Verification items for this drawing (mm, ordinates from the low corner). Round coordinates to 2 decimals unless told otherwise and drop trailing zeros. Order: outer loops, then holes, each group sorted by start corner. A loop starts at its lowest first (then second) coordinate and runs counter-clockwise, first axis right, second up. Notation, with made-up numbers: (49.25, 69) -> (87.25, 69) arc R18 ccw to (87.25, 87) -> close; hole circle Ø3 at (27, -13). An arc over 180 degrees is marked (long way). Answer in a Markdown table with one row per item. Add a question column.
1. Material ranges on L1, parallel to X at y = 48.5, z = 12; L2, parallel to Z at x = 12.25, y = 77.5; L3, parallel to X at y = 8, z = 9.5, recorded low to high. Write a range as from..to.
2. Sectioned sample at A-A, the plane x = 12.7. Record the boundary of the cut face in (y, z) (1 decimal).
3. Depth check by flat-ended pin: P1, Ø5, axis at x = 22, y = 36.5, coming from the -Z side; P2, Ø3, axis at x = 11, y = 64, coming from the +Z side; P3, Ø1, axis at y = 59.5, z = 14, coming from the +X side. Enter the tip coordinate at first touch or a pass-through.
4. Sectioned sample at D-D, the plane z = 20.75. Record the boundary of the cut face in (x, y).
5. Sectioned sample at B-B, the plane z = 12.7. Record the boundary of the cut face in (x, y) (1 decimal).
6. Sectioned sample at C-C, the plane x = 19.75. Record the boundary of the cut face in (y, z) (1 decimal), then the cut area to 3 significant figures.
7. Draft check along Z on the marked faces 1 and 2. Enter one of: +Z half, -Z half, draft (parallel to the pull), parting line (faces both ways), or undercut.
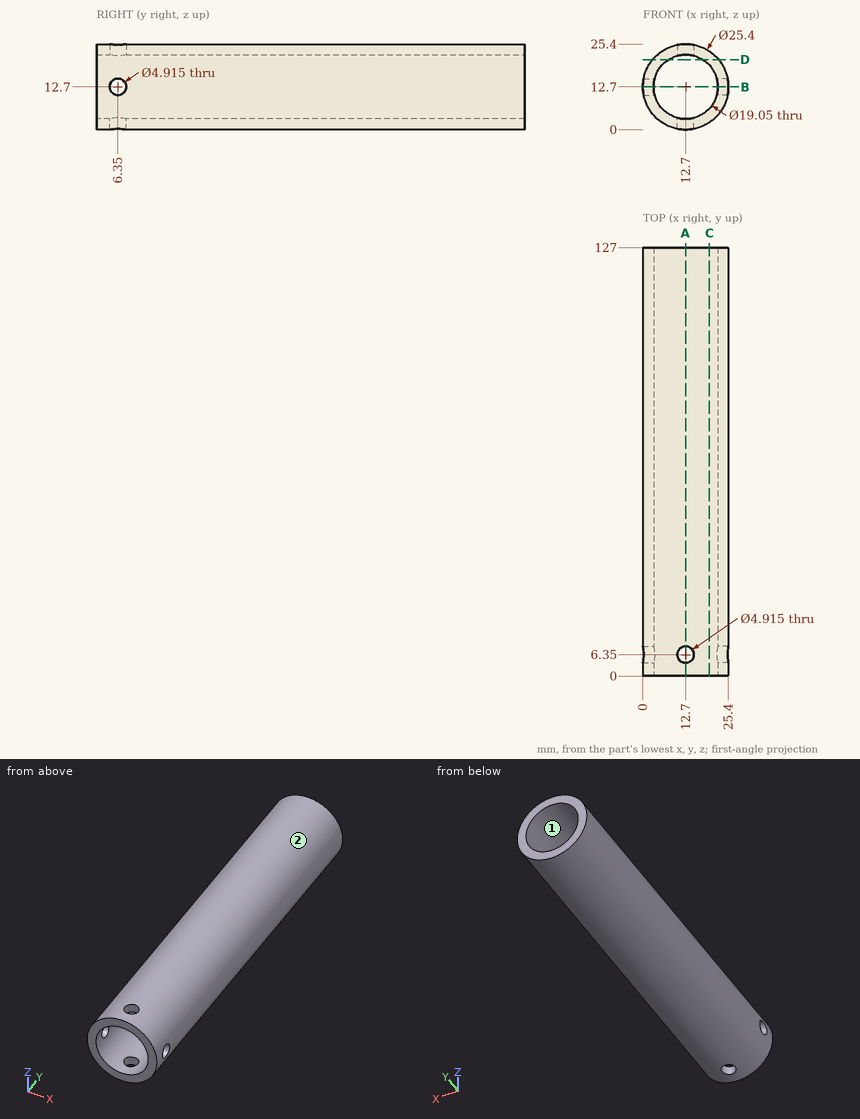
Answer key:
| question | item | result |
|---|---|---|
| 1 | L1 | x = 0.02..3.2, 22.2..25.38 |
| 1 | L2 | z = 0.01..3.19, 22.21..25.39 |
| 1 | L3 | x = 0.41..3.73, 21.67..24.99 |
| 2 | outline | (0, 0) -> (3.9, 0) -> (3.9, 3.2) -> (0, 3.2) -> close; (0, 22.2) -> (3.9, 22.2) -> (3.9, 25.4) -> (0, 25.4) -> close; (8.8, 0) -> (127, 0) -> (127, 3.2) -> (8.8, 3.2) -> close; (8.8, 22.2) -> (127, 22.2) -> (127, 25.4) -> (8.8, 25.4) -> close |
| 3 | P1 | stops at z = 1.97 |
| 3 | P2 | stops at z = 25.4 |
| 3 | P3 | stops at x = 25.37 |
| 4 | outline | (2.88, 0) -> (7.61, 0) -> (7.61, 127) -> (2.88, 127) -> close; (17.79, 0) -> (22.52, 0) -> (22.52, 127) -> (17.79, 127) -> close |
| 5 | outline | (0, 0) -> (3.2, 0) -> (3.2, 3.9) -> (0, 3.9) -> close; (0, 8.8) -> (3.2, 8.8) -> (3.2, 127) -> (0, 127) -> close; (22.2, 0) -> (25.4, 0) -> (25.4, 3.9) -> (22.2, 3.9) -> close; (22.2, 8.8) -> (25.4, 8.8) -> (25.4, 127) -> (22.2, 127) -> close |
| 6 | outline | (0, 2.1) -> (127, 2.1) -> (127, 6.3) -> (0, 6.3) -> close; (0, 19.1) -> (127, 19.1) -> (127, 23.3) -> (0, 23.3) -> close |
| 6 | area | 1,060 mm² |
| 7 | face 1 | undercut |
| 7 | face 2 | parting line |
